```python
from build123d import *

# Parameters (mm, degrees)
EXTRUDE_1_DEPTH     = 6
SKETCH_3_R          = 14
SKETCH_3_R_2        = 11
EXTRUDE_3_DEPTH     = 7
SKETCH_4_R          = 5
CUT_EXTRUDE_1_DEPTH = 87.103712829


with BuildPart() as part:
    # 草图1 → 凸台-拉伸1 (new body)
    with BuildSketch(Plane.XY):
        with BuildLine():
            Line((-26.783524162, 13.993698582), (73.126475838, 10.995048886))
            ThreePointArc((73.126475838, 10.995048886), (83.796475838, 0), (73.126475838, -10.995048886))
            Line((73.126475838, -10.995048886), (-26.783524162, -13.993698582))
            ThreePointArc((-26.783524162, -13.993698582), (-41.203524162, 0), (-26.783524162, 13.993698582))
        make_face()
    extrude(amount=EXTRUDE_1_DEPTH)

    # 草图3 → 凸台-拉伸3 (add, symmetric)
    with BuildSketch(Plane.XY.offset(3)):
        with Locations((-27.203524162, 0)):
            Circle(SKETCH_3_R)
        with Locations((72.796475838, 0)):
            Circle(SKETCH_3_R_2)
    extrude(amount=EXTRUDE_3_DEPTH, both=True)

    # 草图4 → 切除-拉伸1 (cut, through all)
    with BuildSketch(Plane.XY.offset(10)):
        with Locations((72.796475838, 0)):
            Circle(SKETCH_4_R)
        with BuildLine():
            Line((-20.243818708, 0.75), (-17.203524162, 0.75))
            Line((-17.203524162, 0.75), (-17.203524162, -0.75))
            Line((-17.203524162, -0.75), (-20.243818708, -0.75))
            ThreePointArc((-20.243818708, -0.75), (-34.203524162, 0), (-20.243818708, 0.75))
        make_face()
    extrude(amount=-CUT_EXTRUDE_1_DEPTH, mode=Mode.SUBTRACT)


solid = part.part
```
Part model, mm, in its own coordinate system. A direction names the side the tool comes from. Round coordinates to 2 decimals unless told otherwise and drop trailing zeros. Order: outer loops, then holes, each group sorted by start corner. A loop starts at its lowest first (then second) coordinate and runs counter-clockwise, first axis right, second up. Notation, with made-up numbers: M 66,64.5 L 82,64.5 A11 cw 82,78.5 Z; hole C 28.5,88 d10. An arc over 180 degrees is marked long. Answer in a Markdown table with one row per item. Add a question column.
Q1. Wall check: L1, parallel to Z at x = 67, y = -10; L2, parallel to X at y = 1, z = 9; L3, parallel to Y at x = 72.5, z = 2.25. Give the ranges that are in metal, low to high. Write a range as from..to.
Q2. 3-axis set-ups, long thin cutter, end or side, ignore diameter. For faces 3 (the face through (-19, -0.75, 3)), 4 (the face through (78, -2, 10)): which of +Z, -Z, +X, -X, +Y, -Y reach the whole face in a straight line?
Q3. Cut at D-D on x = -6.5. Give the cut face in (y, z).
Q4. Cut at B-B on x = -28. Give the cut face in (y, z).
Q5. Pin check, flat tips, straight feed: pin 1 (1.5 mm diameter, centred on y = -7.5, z = 0.5, fed in from -X); pin 2 (2 mm diameter, centred on x = -9.5, z = -2.5, fed in from +Y); pin 3 (2 mm diameter, centred on x = -19, z = 1.5, fed in from +Y); pin 4 (6 mm diameter, centred on x = 18.5, z = 2, fed in from -Y). Stop position of each tip, or through.
Q6. Cut at C-C on y = 9.25. Give the cut face in (x, z).
Q7. Mould opens along X. For faces 1 (the face through (24, 0, 0)), 2 (the face through (-34, -3, 10)) say: +X half, -X half, draft (parallel to the pull), parting line (faces both ways), or undercut.
Q8. Cut at A-A on z = 1.5. Give the cut face in (x, y).
Established:
| question | item | result |
|---|---|---|
| 1 | L1 | z = 0..6 |
| 1 | L2 | x = -41.17..-34.13, -20.28..-13.24, 61.84..67.9, 77.7..83.75 |
| 1 | L3 | y = -11.01..-4.99, 4.99..11.01 |
| 2 | face 3 | +Z, -Z |
| 2 | face 4 | +Z, +X, -X, +Y, -Y |
| 3 | outline | M -13.38,0 L 13.38,0 L 13.38,6 L -13.38,6 Z |
| 4 | outline | M -13.98,-4 L -6.95,-4 L -6.95,10 L -13.98,10 Z; M 6.95,-4 L 13.98,-4 L 13.98,10 L 6.95,10 Z |
| 5 | pin 1 | stops at x = -39.47 |
| 5 | pin 2 | passes through |
| 5 | pin 3 | stops at y = 13.79 |
| 5 | pin 4 | stops at y = -12.72 |
| 6 | outline | M -37.71,-4 L -16.69,-4 L -16.69,0 L 66.84,0 L 66.84,-4 L 78.75,-4 L 78.75,10 L 66.84,10 L 66.84,6 L -16.69,6 L -16.69,10 L -37.71,10 Z |
| 7 | face 1 | undercut |
| 7 | face 2 | draft |
| 8 | outline | M -26.78,-13.99 L 73.13,-11 A11 ccw 73.13,11 L -26.78,13.99 A14 ccw long Z; hole M -20.24,-0.75 L -17.2,-0.75 L -17.2,0.75 L -20.24,0.75 A7 ccw long Z; hole C 72.8,0 d10 |
